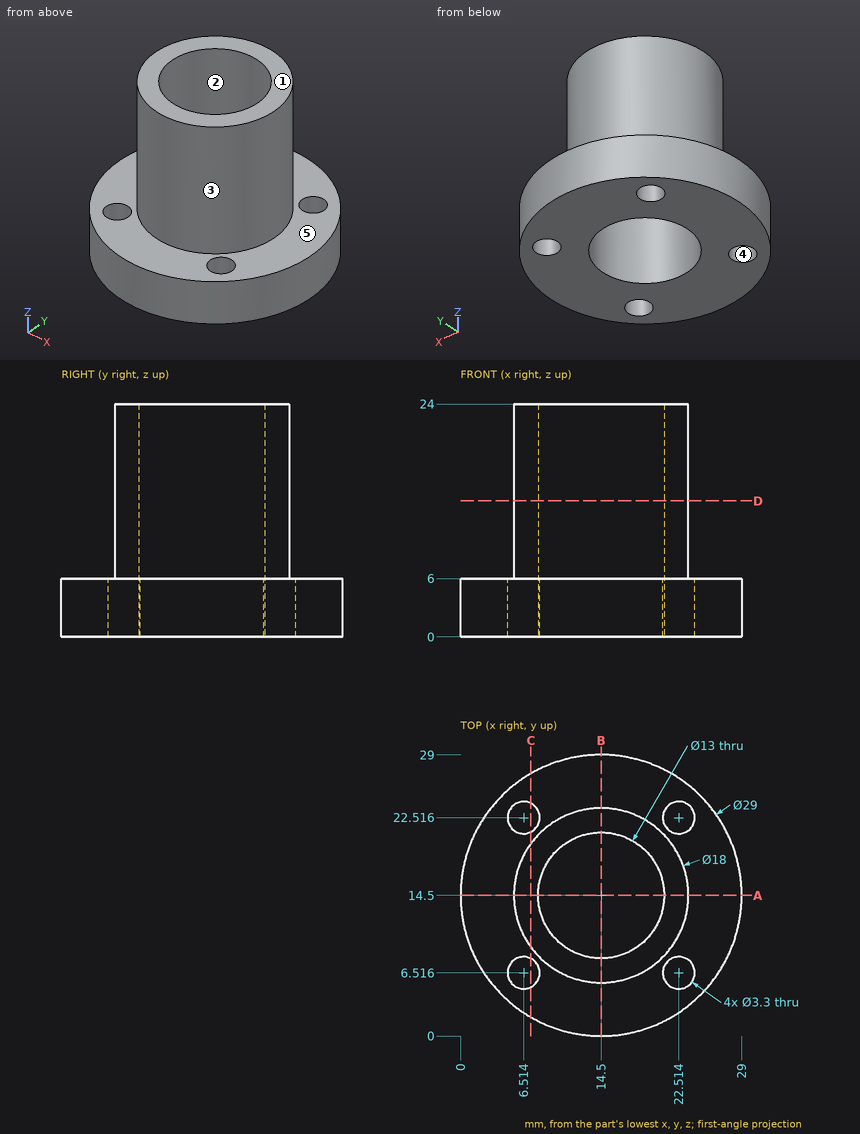
The drawing under review shows one solid part. Ordinate dimensions are in mm from its lowest x, y, z. A direction names the side the tool comes from. Give positions to 0.01 mm unless a question says otherwise; leave off trailing zeros. Write each loop counter-clockwise with the first axis right and the second up, starting at its lowest first coordinate (ties: lowest second). Pieces come first, ordered by that corner, then holes. Notation, with made-up numbers: (-29, 83) -> (-7, 83) arc R14 cw to (-7, 101) -> close; hole circle Ø9 at (-22, 36). An arc over 180 degrees is marked (long way). Use CSV: the item, a comma, the result in double quotes.
Q1. Tool access review of the marked faces 4 and 5: name each direction out of +Z, -Z, +X, -X, +Y, -Y from which nothing blocks a thin tool from reaching the whole face with its end or side.
Conclusion:
face 4,"+Z, -Z"
face 5,"+Z"
Q2. For P1, Ø4.5, axis at x = 6.51, y = 22.52, coming from the +Z side; P2, Ø12, axis at y = 12, z = 15, coming from the +X side; P3, Ø10, axis at x = 20, z = 14, coming from the -Y side, all flat-tipped, find the tip position at first contact; note any pin that passes through.
Conclusion:
P1,"z = 6"
P2,"x = 23.5"
P3,"y = 5.51"
Q3. Take a section at A-A, the plane y = 14.5. Write out the cut boundary in (x, z).
Conclusion:
outline,"(0, 0) -> (8, 0) -> (8, 24) -> (5.5, 24) -> (5.5, 6) -> (0, 6) -> close; (21, 0) -> (29, 0) -> (29, 6) -> (23.5, 6) -> (23.5, 24) -> (21, 24) -> close"
Q4. Take a section at D-D, the plane z = 14. Write out the cut boundary in (x, y), then the cut area to 3 significant figures.
Conclusion:
outline,"circle Ø18 at (14.5, 14.5); hole circle Ø13 at (14.5, 14.5)"
area,"122 mm2"
Q5. To check wall thickness, follow probe 1 along X at (y, z) = (23.25, 2.25) (1 decimal); probe 2 along Y at (x, z) = (23.25, 1); probe 3 along X at (y, z) = (14, 11). State the ranges of each line that lie inside material, in increasing order. Write a range as [from, to].
Conclusion:
probe 1,"[2.9, 5], [8, 21], [24, 26.1]"
probe 2,"[2.94, 5.04], [7.99, 21.04], [23.99, 26.06]"
probe 3,"[5.51, 8.02], [20.98, 23.49]"
Q6. Mouldability with a two-part tool opening along Y and no side actions: class the marked faces 1, 2 and 3 as pulls with the +Y half, pulls with the -Y half, needs draft (parallel to the pull), parting line crosses it, or undercut.
Conclusion:
face 1,"needs draft"
face 2,"undercut"
face 3,"parting line crosses it"
Q7. Take a section at C-C, the plane x = 7.25. Write out the cut boundary in (y, z), then the cut area to 3 significant figures.
Conclusion:
outline,"(1.94, 0) -> (5.04, 0) -> (5.04, 6) -> (1.94, 6) -> close; (7.99, 0) -> (21.04, 0) -> (21.04, 6) -> (19.83, 6) -> (19.83, 24) -> (9.17, 24) -> (9.17, 6) -> (7.99, 6) -> close; (23.99, 0) -> (27.06, 0) -> (27.06, 6) -> (23.99, 6) -> close"
area,"307 mm2"
